from build123d import *

# Parameters (mm, degrees)
F0_W     = 38.1
F0_H     = 25.4
F1_DEPTH = 50.8
F2_W     = 34.29
F2_H     = 48.895
F3_DEPTH = 25.4
F4_R     = 10.16
F5_DEPTH = 50.8


with BuildPart() as f1:
    # F0 (on Top) → F1 (new body)
    with BuildSketch(Plane.XY):
        with Locations((19.05, 12.7)):
            Rectangle(F0_W, F0_H)
    extrude(amount=F1_DEPTH)

    # F2 (on face) → F3 (cut)
    with BuildSketch(Plane.XZ):
        with Locations((19.05, 26.3525)):
            Rectangle(F2_W, F2_H)
    extrude(amount=-F3_DEPTH, mode=Mode.SUBTRACT)

    # F4 (on face) → F5 (cut)
    with BuildSketch(Plane.YZ.offset(38.1)):
        with Locations((12.7, 39.37)):
            Circle(F4_R)
        with Locations((12.7, 13.97)):
            Circle(F4_R)
    extrude(amount=-F5_DEPTH, mode=Mode.SUBTRACT)


solid = f1.part
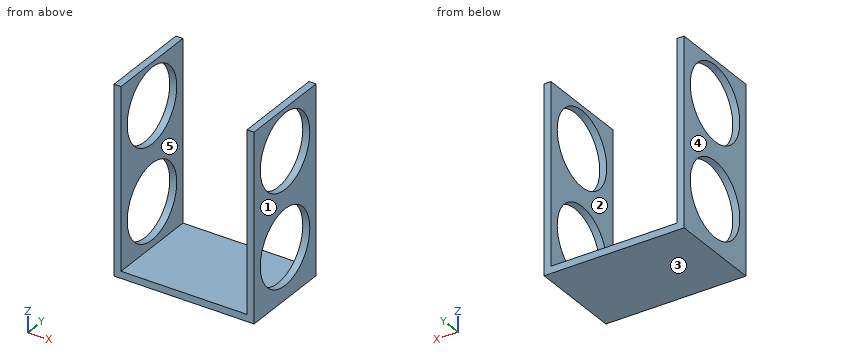
Geometry check sheet. Reference: the model listing, model coordinates, mm. Face numbers are marked on the shaded views. A direction names the side the tool comes from. Round coordinates to 2 decimals unless told otherwise and drop trailing zeros. Write each loop counter-clockwise with the first axis right and the second up, starting at its lowest first coordinate (ties: lowest second). Pieces come first, ordered by that corner, then holes. Notation, with made-up numbers: (-16, 63) -> (4, 63) arc R30 ccw to (4, 90) -> close; hole circle Ø4 at (12.25, 41). An arc over 180 degrees is marked (long way). One line per item, written item: value. Start each with the question number.
(1) Cross-section at C-C, the plane z = 26.5. Record the cut outline in (x, y) (3 decimals), and give its area (3 significant figures).
(2) Access from +Z, -Z, +X, -X, +Y, -Y to the whole of each face (thin tool, end or side, straight path). Record for the marked faces 1 and 2.
(3) Cross-section at D-D, the plane x = 10.5. Record the cut outline in (y, z) (3 decimals), and give its area (3 significant figures).
(4) Draft check along X on the marked faces 3, 4 and 5. Enter one of: +X half, -X half, draft (parallel to the pull), parting line (faces both ways), or undercut.
(5) Cross-section at B-B, the plane y = 12.7. Record the cut outline in (x, z) (3 decimals), and give its area (3 significant figures).
(6) Scan lines: line 1 (Z direction, x = 0.5, y = 12.7); line 2 (X direction, y = 21.25, z = 30) (3 decimals); line 3 (Z direction, x = 19.5, y = 16.75) (3 decimals). Record each from-to range of solid material in increasing order. Write a range as [from, to].
(7) Go/stop test with flat-tipped pins: pin 1 Ø12.5 at (x, y) = (11.5, 6.5) entering from +Z (3 decimals); pin 2 Ø12 at (y, z) = (12.7, 13.97) entering from -X. Record where each tip stops, or that it passes through.
(8) Cross-section at A-A, the plane z = 39.37. Record the cut outline in (x, y) (3 decimals), and give its area (3 significant figures).
Answer:
1. outline: (0, 0) -> (1.905, 0) -> (1.905, 25.4) -> (0, 25.4) -> close; (36.195, 0) -> (38.1, 0) -> (38.1, 25.4) -> (36.195, 25.4) -> close
1. area: 96.8 mm²
2. face 1: +Z, -Z, +X, +Y, -Y
2. face 2: +Z, +Y, -Y
3. outline: (0, 0) -> (25.4, 0) -> (25.4, 1.905) -> (0, 1.905) -> close
3. area: 48.4 mm²
4. face 3: draft
4. face 4: -X half
4. face 5: undercut
5. outline: (0, 0) -> (38.1, 0) -> (38.1, 3.81) -> (36.195, 3.81) -> (36.195, 1.905) -> (1.905, 1.905) -> (1.905, 3.81) -> (0, 3.81) -> close; (0, 24.13) -> (1.905, 24.13) -> (1.905, 29.21) -> (0, 29.21) -> close; (0, 49.53) -> (1.905, 49.53) -> (1.905, 50.8) -> (0, 50.8) -> close; (36.195, 24.13) -> (38.1, 24.13) -> (38.1, 29.21) -> (36.195, 29.21) -> close; (36.195, 49.53) -> (38.1, 49.53) -> (38.1, 50.8) -> (36.195, 50.8) -> close
5. area: 104 mm²
6. line 1: [0, 3.81], [24.13, 29.21], [49.53, 50.8]
6. line 2: [0, 1.905], [36.195, 38.1]
6. line 3: [0, 1.905]
7. pin 1: z = 1.905
7. pin 2: through
8. outline: (0, 0) -> (1.905, 0) -> (1.905, 2.54) -> (0, 2.54) -> close; (0, 22.86) -> (1.905, 22.86) -> (1.905, 25.4) -> (0, 25.4) -> close; (36.195, 0) -> (38.1, 0) -> (38.1, 2.54) -> (36.195, 2.54) -> close; (36.195, 22.86) -> (38.1, 22.86) -> (38.1, 25.4) -> (36.195, 25.4) -> close
8. area: 19.4 mm²
